```python
from build123d import *

# Parameters (mm, degrees)
SKETCH1_R           = 10
BOSS_EXTRUDE1_DEPTH = 5
BOSS_EXTRUDE2_DEPTH = 2
BOSS_EXTRUDE3_REACH = 39.189
SKETCH3_W           = 2
SKETCH3_H           = 2
BOSS_EXTRUDE5_DEPTH = 2
FILLET1_R           = 2


with BuildPart() as part:
    # Sketch1 → Boss-Extrude1 (new body)
    with BuildSketch(Plane(origin=(0, 0, 0), x_dir=(1, 0, 0), z_dir=(0, 1, 0))):
        with Locations(Location((0, 0, 0), (0, 0, 270))):
            Circle(SKETCH1_R)
        with BuildLine():
            Line((-1.25, -1.224744871), (-1.25, 1.224744871))
            ThreePointArc((-1.25, 1.224744871), (1.75, 0), (-1.25, -1.224744871))
        make_face(mode=Mode.SUBTRACT)
    extrude(amount=BOSS_EXTRUDE1_DEPTH)

    # Sketch2 → Boss-Extrude2 (add)
    with BuildSketch(Plane(origin=(0, 5, 0), x_dir=(1, 0, 0), z_dir=(0, 1, 0))):
        Polygon((8.660254038, 5), (33.660254038, 5), (33.660254038, 7), (7.141428429, 7), align=None)
        Polygon((7.141428429, -7), (33.660254038, -7), (33.660254038, -5), (8.660254038, -5), align=None)
    extrude(amount=-BOSS_EXTRUDE2_DEPTH)

    # Sketch3 → Boss-Extrude3 (add, up to next)
    with BuildSketch(Plane(origin=(0, 0, 5), x_dir=(-1, 0, 0), z_dir=(0, 0, -1)), mode=Mode.PRIVATE) as boss_extrude3_sk1:
        with Locations((-32.660254038, 4)):
            Rectangle(SKETCH3_W, SKETCH3_H)
    boss_extrude3_tool1 = extrude(boss_extrude3_sk1.sketch, amount=BOSS_EXTRUDE3_REACH, mode=Mode.PRIVATE) - part.part
    add(boss_extrude3_tool1.solids().sort_by_distance((32.660254, 4, 5))[0])

    # Sketch4 → Boss-Extrude5 (add)
    with BuildSketch(Plane(origin=(0, 5, 0), x_dir=(1, 0, 0), z_dir=(0, 1, 0))):
        Polygon((11.488681163, -5), (15.0744676, -1.414213562), (18.660254038, -5), (21.488681163, -5), (16.488681163, 0), (21.488681163, 5), (18.660254038, 5), (15.0744676, 1.414213562), (11.488681163, 5), (8.660254038, 5), (13.660254038, 0), (8.660254038, -5), align=None)
    extrude(amount=-BOSS_EXTRUDE5_DEPTH)

    # Fillet1
    fillet1_edges = [part.edges().sort_by_distance(p)[0] for p in [
        (33.660254038, 4, -7),
        (33.660254038, 4, 7),
        (31.660254038, 4, -5),
        (31.660254038, 4, 5),
    ]]
    fillet(fillet1_edges, radius=FILLET1_R)


solid = part.part
```
The listing builds one solid part. Answer for the finished solid, in the listing's coordinates (mm). A direction names the side the tool comes from. Round coordinates to 2 decimals unless told otherwise and drop trailing zeros. Loops run counter-clockwise (first coordinate to the right, second up) from the corner with the lowest first, then second, coordinate; pieces in that order, holes last.
Q1. For a pull along Z with two mould halves and no side action, classify faces 1 (the face through (33.09, 3.99, -6.4)), 2 (the face through (19, 4, 7)), 3 (the face through (16.84, 4.01, 3.18)), 4 (the face through (7, 5, 0)) as released by +Z, released by -Z, zero draft, split by the parting line, or undercut.
Q2. Find the intervals of material crossed by line 1 (X direction, y = 1.65, z = 0); line 2 (Z direction, x = 12, y = 4.7); line 3 (X direction, y = 3.45, z = -4.5), in increasing order.
Q3. Given pin 1 Ø1.6 at (x, y) = (15, 3.5) entering from -Z; pin 2 Ø2 at (y, z) = (4, -3) entering from -X; pin 3 Ø0.6 at (x, y) = (27, 4) entering from +Z; pin 4 Ø1 at (x, y) = (23, 1) entering from -Z, each flat-ended and moving along its own axis, determine where each tip first touches the part or whether it passes through.
Q4. Section D-D, the plane y = 1.1 is taken. Determine the outline of the cut face in (x, z), then the cut area to 3 significant figures.
Q5. Section C-C, the plane x = 8 is taken. Determine the outline of the cut face in (y, z), then the cut area to 3 significant figures.
Q6. Section B-B, the plane y = 3.6 is taken. Determine the outline of the cut face in (x, z).
Q7. Which of the six approach directions +Z, -Z, +X, -X, +Y, -Y give full straight-line access (tool end or side, diameter ignored) to faces 5 (the face through (33.66, 4, 0)), 6 (the face through (15, 4, 5))?
Q8. Section A-A, the plane x = 0 is taken. Determine the outline of the cut face in (y, z), then the cut area to 3 significant figures.
Completed:
1. face 1: released by -Z
1. face 2: released by +Z
1. face 3: undercut
1. face 4: zero draft
2. line 1: x = -10 to -1.25, 1.75 to 10
2. line 2: z = -7 to -5, -4.49 to -1.66, 1.66 to 4.49, 5 to 7
2. line 3: x = -8.93 to 8.93, 9.16 to 11.99, 18.16 to 20.99, 30.98 to 33.66
3. pin 1: stops at z = -7
3. pin 2: stops at x = -9.8
3. pin 3: stops at z = 7
3. pin 4: passes through
4. outline: circle Ø20 at (0, 0); hole (-1.25, -1.22) arc R1.75 ccw (long way) to (-1.25, 1.22) - close
4. area: 305 mm2
5. outline: (0, -6) - (3, -6) - (3, -7) - (5, -7) - (5, 7) - (3, 7) - (3, 6) - (0, 6) - close
5. area: 64.0 mm2
6. outline: (7.14, -7) - (31.66, -7) arc R2 ccw to (33.66, -5) - (33.66, 5) arc R2 ccw to (31.66, 7) - (7.14, 7) arc R10 ccw (long way) to start; hole (-1.25, -1.22) arc R1.75 ccw (long way) to (-1.25, 1.22) - close; hole (8.66, -5) - (13.66, 0) - (8.66, 5) arc R10 cw to start; hole (11.49, -5) - (18.66, -5) - (15.07, -1.41) - close; hole (11.49, 5) - (15.07, 1.41) - (18.66, 5) - close; hole (16.49, 0) - (21.49, -5) - (29.66, -5) arc R2 ccw to (31.66, -3) - (31.66, 3) arc R2 ccw to (29.66, 5) - (21.49, 5) - close
7. face 5: +Z, -Z, +X, +Y, -Y
7. face 6: +Y, -Y
8. outline: (0, -10) - (5, -10) - (5, -1.75) - (0, -1.75) - close; (0, 1.75) - (5, 1.75) - (5, 10) - (0, 10) - close
8. area: 82.5 mm2
